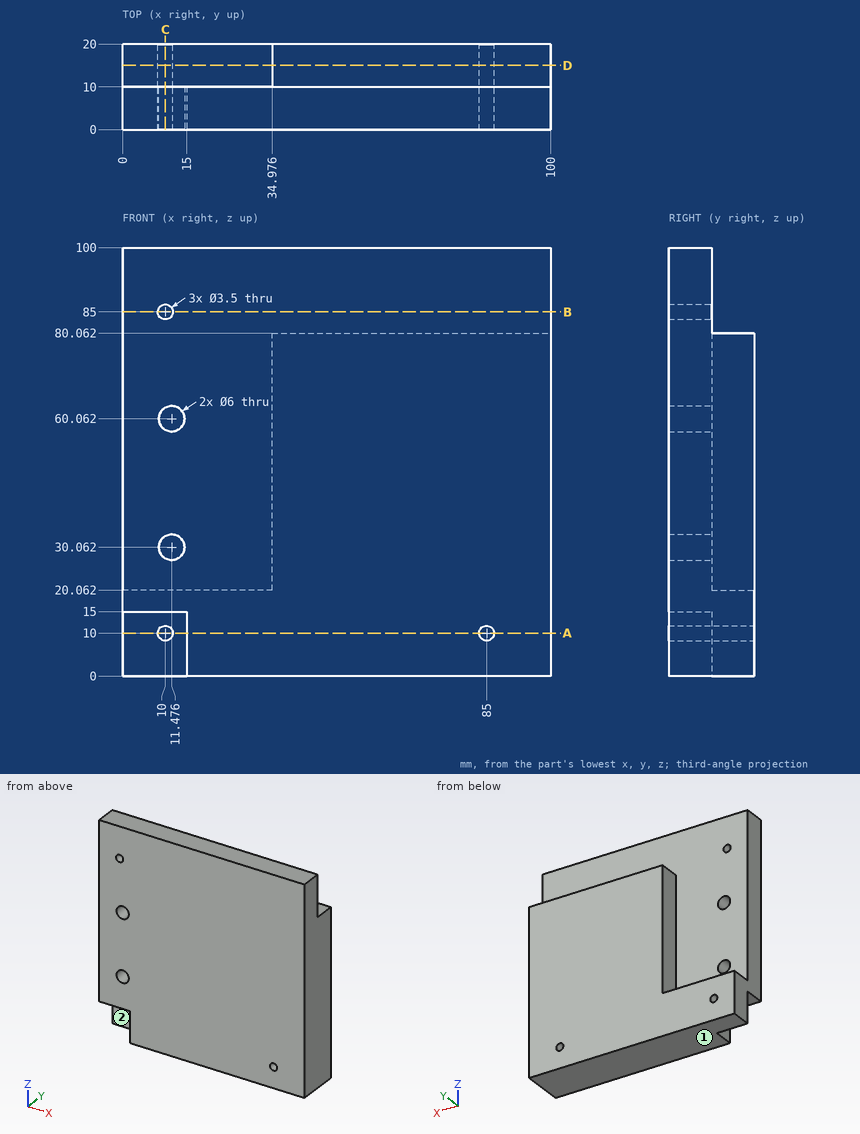
Design review of the part shown in the three views and the two pictorial views. Dimensions are in mm from the part's minimum x, y and z. A direction names the side the tool comes from. Coordinates: 2 decimals unless noted, no trailing zeros. Loops run counter-clockwise (first coordinate to the right, second up) from the corner with the lowest first, then second, coordinate; pieces in that order, holes last. Notation, with made-up numbers: (74, -34.5) - (119, -34.5) arc R29 ccw to (119, -0.5) - close; hole circle Ø1 at (48, -1). An arc over 180 degrees is marked (long way). Use a Markdown table: item, result. Add a question column.
Item 1: We need section C-C (x = 10). Give the boundary of the cut face in (y, z).
Item 2: We need section D-D (y = 15). Give the boundary of the cut face in (x, z).
Item 3: Insertion check: pin 1 Ø1.5 at (x, y) = (82.5, 10.5) entering from -Z; pin 2 Ø3 at (x, y) = (24, 15) entering from +Z; pin 3 Ø8 at (x, y) = (5, 4) entering from -Z; pin 4 Ø2 at (x, z) = (10, 85) entering from -Y. Each pin has a flat end and moves straight along its axis. Give the tip position at first contact, or say it passes through.
Item 4: Tool access review of the marked faces 1 and 2: name each direction out of +Z, -Z, +X, -X, +Y, -Y from which nothing blocks a thin tool from reaching the whole face with its end or side.
Item 5: We need section B-B (z = 85). Give the boundary of the cut face in (x, y), and give its area (3 significant figures).
Item 6: We need section A-A (z = 10). Give the boundary of the cut face in (x, y), and give its area (4 significant figures).
Item 7: For line 1 (X direction, y = 14, z = 10); line 2 (Z direction, x = 85, y = 14.25); line 3 (X direction, y = 6.5, z = 10), list the stretches that pass through material, from the lowest coordinate up.
Results list:
| question | item | result |
|---|---|---|
| 1 | outline | (0, 15) - (10, 15) - (10, 11.75) - (20, 11.75) - (20, 20.06) - (10, 20.06) - (10, 27.45) - (0, 27.45) - close; (0, 32.67) - (10, 32.67) - (10, 57.45) - (0, 57.45) - close; (0, 62.67) - (10, 62.67) - (10, 83.25) - (0, 83.25) - close; (0, 86.75) - (10, 86.75) - (10, 100) - (0, 100) - close; (10, 0) - (20, 0) - (20, 8.25) - (10, 8.25) - close |
| 2 | outline | (0, 0) - (100, 0) - (100, 80.06) - (34.98, 80.06) - (34.98, 20.06) - (0, 20.06) - close; hole circle Ø3.5 at (10, 10); hole circle Ø3.5 at (85, 10) |
| 3 | pin 1 | stops at z = 0 |
| 3 | pin 2 | stops at z = 20.06 |
| 3 | pin 3 | stops at z = 15 |
| 3 | pin 4 | passes through |
| 4 | face 1 | -Z, +X, -X, +Y, -Y |
| 4 | face 2 | -Z, -X, -Y |
| 5 | outline | (0, 0) - (8.25, 0) - (8.25, 10) - (0, 10) - close; (11.75, 0) - (100, 0) - (100, 10) - (11.75, 10) - close |
| 5 | area | 965 mm^2 |
| 6 | outline | (0, 10) - (8.25, 10) - (8.25, 20) - (0, 20) - close; (11.75, 10) - (15, 10) - (15, 0) - (83.25, 0) - (83.25, 20) - (11.75, 20) - close; (86.75, 0) - (100, 0) - (100, 20) - (86.75, 20) - close |
| 6 | area | 1,745 mm^2 |
| 7 | line 1 | x = 0 to 8.25, 11.75 to 83.25, 86.75 to 100 |
| 7 | line 2 | z = 0 to 8.25, 11.75 to 80.06 |
| 7 | line 3 | x = 15 to 83.25, 86.75 to 100 |
